```python
from build123d import *

# Parameters (mm, degrees)
SKETCH_1_W          = 15
SKETCH_1_H          = 30
EXTRUDE_1_DEPTH     = 2
EXTRUDE_2_DEPTH     = 10
FILLET_1_R          = 1.5
SKETCH_3_W          = 10
SKETCH_3_H          = 17
CUT_EXTRUDE_1_DEPTH = 3
SKETCH_4_W          = 55
SKETCH_4_H          = 30
EXTRUDE_3_DEPTH     = 2
SKETCH_5_W          = 47
SKETCH_5_H          = 14
EXTRUDE_4_DEPTH     = 2
SKETCH_6_W          = 2
SKETCH_6_H          = 5
EXTRUDE_5_DEPTH     = 14
EXTRUDE_6_DEPTH     = 12
EXTRUDE_7_DEPTH     = 31
FILLET_4_R          = 3


with BuildPart() as part:
    # Sketch 1 → Extrude 1 (new body)
    with BuildSketch(Plane.XY):
        Rectangle(SKETCH_1_W, SKETCH_1_H)
    extrude(amount=EXTRUDE_1_DEPTH)

    # Sketch 2 → Extrude 2 (add)
    with BuildSketch(Plane(origin=(5.5, 0, 0), x_dir=(0, 0, -1), z_dir=(1, 0, 0))):
        Polygon((-2, 10), (-8, 10), (-8, -10), (-2, -10), (-2, -8.5), (-6.5, -8.5), (-6.5, 8.5), (-2, 8.5), align=None)
    extrude(amount=-EXTRUDE_2_DEPTH)

    # Fillet 1
    fillet_1_edges = [part.edges().sort_by_distance(p)[0] for p in [
        (0.5, 8.5, 6.5),
        (0.5, -8.5, 6.5),
    ]]
    fillet(fillet_1_edges, radius=FILLET_1_R)

    # Sketch 3 → Cut-Extrude 1 (cut)
    with BuildSketch(Plane(origin=(0, 0, 0), x_dir=(-1, 0, 0), z_dir=(0, 0, -1))):
        with Locations((-0.5, 0)):
            Rectangle(SKETCH_3_W, SKETCH_3_H)
    extrude(amount=-CUT_EXTRUDE_1_DEPTH, mode=Mode.SUBTRACT)

    # Sketch 5 → Extrude 4 (add)
    with BuildSketch(Plane(origin=(0, 0, 6.5), x_dir=(-1, 0, 0), z_dir=(0, 0, -1))):
        with Locations((-21, 0)):
            Rectangle(SKETCH_5_W, SKETCH_5_H)
    extrude(amount=EXTRUDE_4_DEPTH)

    # Sketch 6 → Extrude 5 (add)
    with BuildSketch(Plane.XZ.offset(7)):
        with Locations((28.5, 9)):
            Rectangle(SKETCH_6_W, SKETCH_6_H)
    extrude(amount=-EXTRUDE_5_DEPTH)



with BuildPart() as body_2:
    # Sketch 4 → Extrude 3 (new body)
    with BuildSketch(Plane.XY.offset(2)):
        with Locations((43, 0)):
            Rectangle(SKETCH_4_W, SKETCH_4_H)
    extrude(amount=-EXTRUDE_3_DEPTH)


with BuildPart() as part_1:
    add(part.part)

    add(body_2.part)  # Extrude 6 merges body 2
    # Sketch 7 → Extrude 6 (add)
    with BuildSketch(Plane.ZY.offset(-15.5)):
        with BuildLine():
            Line((6.5, -7), (6.5, 7))
            ThreePointArc((6.5, 7), (6.060660172, 8.060660172), (5, 8.5))
            Line((5, 8.5), (2, 8.5))
            Line((2, 8.5), (2, 10))
            Line((2, 10), (8, 10))
            Line((8, 10), (8, -10))
            Line((8, -10), (2, -10))
            Line((2, -10), (2, -8.5))
            Line((2, -8.5), (5, -8.5))
            ThreePointArc((5, -8.5), (6.060660172, -8.060660172), (6.5, -7))
        make_face()
    extrude(amount=-EXTRUDE_6_DEPTH)

    # Sketch 8 → Extrude 7 (add)
    with BuildSketch(Plane(origin=(39.5, 0, 0), x_dir=(0, 0, -1), z_dir=(1, 0, 0))):
        with BuildLine():
            Line((-6.5, 7), (-6.5, -7))
            ThreePointArc((-6.5, -7), (-6.060660172, -8.060660172), (-5, -8.5))
            Line((-5, -8.5), (-2, -8.5))
            Line((-2, -8.5), (-2, -10))
            Line((-2, -10), (-8, -10))
            Line((-8, -10), (-8, 10))
            Line((-8, 10), (-2, 10))
            Line((-2, 10), (-2, 8.5))
            Line((-2, 8.5), (-5, 8.5))
            ThreePointArc((-5, 8.5), (-6.060660172, 8.060660172), (-6.5, 7))
        make_face()
    extrude(amount=EXTRUDE_7_DEPTH)

    # Fillet 4
    fillet_4_edges = [part_1.edges().sort_by_distance(p)[0] for p in [
        (-7.5, -15, 1),
        (-7.5, 15, 1),
        (7.5, 15, 1),
        (15.5, 15, 1),
        (70.5, 15, 1),
        (7.5, -15, 1),
        (15.5, -15, 1),
        (70.5, -15, 1),
        (28.5, -7, 11.5),
        (28.5, 7, 11.5),
        (55, 10, 8),
        (55, -10, 8),
        (21.5, -10, 8),
        (21.5, 10, 8),
        (0.5, -10, 8),
        (0.5, 10, 8),
    ]]
    fillet(fillet_4_edges, radius=FILLET_4_R)


solid = part_1.part
```
CAD build for the part. Positions are in the model's coordinates, mm. A direction names the side the tool comes from. Give positions to 0.01 mm unless a question says otherwise; leave off trailing zeros. Write each loop counter-clockwise with the first axis right and the second up, starting at its lowest first coordinate (ties: lowest second). Pieces come first, ordered by that corner, then holes. Notation, with made-up numbers: M -9.75,28 L 11.25,28 A20 cw 11.25,52 Z; hole C 76,3 d7. An arc over 180 degrees is marked long. Return JSON: item names as keys, results as strings. Group by question number.
(1) Band-saw the part on C-C (x = 33). Give the cut face in (y, z), and give its area (3 significant figures).
(2) Flat gauge pins, fed straight in: pin 1 Ø1 at (x, y) = (58.5, 11.5) entering from +Z; pin 2 Ø1 at (x, y) = (-3.5, 2.5) entering from -Z; pin 3 Ø1 at (x, y) = (61, -8.5) entering from -Z; pin 4 Ø5 at (x, y) = (-1, -1) entering from +Z. Where does each tip first touch, or does it go through?
(3) Mould opens along Z. For faces 1 (the face through (28.51, 6.14, 10.6)), 2 (the face through (21, 8.5, 4)), 3 (the face through (-4.5, 0, 1)) say: pulls with the +Z half, pulls with the -Z half, needs draft (parallel to the pull), parting line crosses it, or undercut.
(4) 3-axis set-ups, long thin cutter, end or side, ignore diameter. For faces 4 (the face through (21, -10, 4)), 5 (the face through (21, 0, 4.5)), 6 (the face through (29.5, 0, 9)), 7 (the face through (16.4, -14.14, 0.99)): which of +Z, -Z, +X, -X, +Y, -Y reach the whole face in a straight line?
(5) Band-saw the part on D-D (y = -11). Give the cut face in (x, z), and give its area (3 significant figures).
(6) Band-saw the part on B-B (y = -5.5). State how many separate pieces and enclosed holes the cut face has, and give its area (3 significant figures).
(7) Drill centre lines: L1, parallel to Y at x = 3, z = 0.5; L2, parallel to Z at x = 34.5, y = -6.5; L3, parallel to Y at x = 23, z = 4.25. Where is each one in solid material? Low to high. Write a range as [from, to].
(8) Band-saw the part on A-A (x = 64). Give the cut face in (y, z).
Entries:
{
 "1": {"outline": "M -15,0 L 15,0 L 15,2 L -15,2 Z; M -7,4.5 L 7,4.5 L 7,6.5 L -7,6.5 Z", "area": "88.0 mm^2"},
 "2": {"pin 1": "stops at z = 2", "pin 2": "stops at z = 6.5", "pin 3": "stops at z = 0", "pin 4": "stops at z = 8"},
 "3": {"face 1": "pulls with the +Z half", "face 2": "undercut", "face 3": "needs draft"},
 "4": {"face 4": "+Z, +X, -X, -Y", "face 5": "+X, -X", "face 6": "+Z, +Y, -Y", "face 7": "+Z, -Z, -Y"},
 "5": {"outline": "M -7.5,0 L 7.5,0 L 7.5,2 L -7.5,2 Z; M 15.5,0 L 70.5,0 L 70.5,2 L 15.5,2 Z", "area": "140 mm^2"},
 "6": {"separate pieces": "4", "enclosed holes": "0", "area": "303 mm^2"},
 "7": {"L1": "y = [-15, -8.5], [8.5, 15]", "L2": "z = [0, 2], [4.5, 6.5]", "L3": "y = [-10, -8.5], [8.5, 10]"},
 "8": {"outline": "M -15,0 L 15,0 L 15,2 L 10,2 L 10,5 A3 ccw 7,8 L -7,8 A3 ccw -10,5 L -10,2 L -15,2 Z; hole M -8.5,2 L 8.5,2 L 8.5,5 A1.5 ccw 7,6.5 L -7,6.5 A1.5 ccw -8.5,5 Z"}
}
